from build123d import *

# Parameters (mm, degrees)
SKETCH1_W           = 15
SKETCH1_H           = 15
BOSS_EXTRUDE1_DEPTH = 10
BOSS_EXTRUDE2_DEPTH = 1.5


with BuildPart() as part:
    # Sketch1 → Boss-Extrude1 (new body)
    with BuildSketch(Plane.XY):
        with Locations((7.5, -7.5)):
            Rectangle(SKETCH1_W, SKETCH1_H)
    extrude(amount=BOSS_EXTRUDE1_DEPTH)

    # Sketch2 → Boss-Extrude2 (add, symmetric)
    with BuildSketch(Plane(origin=(7.5, 0, 0), x_dir=(0, 0, -1), z_dir=(1, 0, 0))):
        with BuildLine():
            ThreePointArc((3, -5), (0.5, -7.5), (3, -10))
            Line((3, -10), (3, -8.5))
            ThreePointArc((3, -8.5), (2, -7.5), (3, -6.5))
            Line((3, -6.5), (3, -5))
        make_face()
        with BuildLine():
            Line((3, -8.5), (3, -10))
            ThreePointArc((3, -10), (4.767766953, -9.267766953), (5.5, -7.5))
            ThreePointArc((5.5, -7.5), (4.767766953, -5.732233047), (3, -5))
            Line((3, -5), (3, -6.5))
            ThreePointArc((3, -6.5), (3.707106781, -6.792893219), (4, -7.5))
            ThreePointArc((4, -7.5), (3.707106781, -8.207106781), (3, -8.5))
        make_face()
        with BuildLine():
            Line((0, -10), (3, -10))
            ThreePointArc((3, -10), (0.5, -7.5), (3, -5))
            Line((3, -5), (0, -5))
            Line((0, -5), (0, -10))
        make_face()
    extrude(amount=BOSS_EXTRUDE2_DEPTH, both=True)


solid = part.part
Check sheet for the modelled part. Datum: model origin and axes. Units: mm. A direction names the side the tool comes from. Round coordinates to 2 decimals unless told otherwise and drop trailing zeros. Loops run counter-clockwise (first coordinate to the right, second up) from the corner with the lowest first, then second, coordinate; pieces in that order, holes last. Notation, with made-up numbers: (-9.75, 19.25) - (1.25, 19.25) arc R7 ccw to (1.25, 27.25) - close; hole circle Ø11 at (8.25, -9.5). An arc over 180 degrees is marked (long way). Answer as CSV lines item,"result". Start each with the question number.
Item 1: Section check B-B (z = -2.75). Record the boundary of the cut face in (x, y).
Item 2: Section check D-D (y = -14). Record the boundary of the cut face in (x, z).
Item 3: Section check A-A (x = 8.5). Record the boundary of the cut face in (y, z).
Item 4: Scan lines: line 1 (Z direction, x = 13.75, y = -4.75); line 2 (Y direction, x = 8, z = -2.5). Record each from-to range of solid material in increasing order. Write a range as [from, to].
Item 5: Section check C-C (y = -6.75). Record the boundary of the cut face in (x, z).
Item 6: Set-up check for faces 1 (the flat face through (9, -7, -1)), 2 (the flat face through (6, -7, -1)), 3 (the flat face through (8, -5, -2)), 4 (the flat face through (8, -10, -1)): record each of +Z, -Z, +X, -X, +Y, -Y from which the full face is reachable in a straight line by a thin tool's end or side.
Item 7: Depth check by flat-ended pin: P1, Ø1.5, axis at x = 7.5, z = -1, coming from the -Y side; P2, Ø6, axis at y = -6.5, z = -0.5, coming from the -X side; P3, Ø5.5, axis at y = -8, z = -4, coming from the -X side; P4, Ø2.5, axis at x = 7, z = -1.5, coming from the +Y side. Enter the tip coordinate at first touch or a pass-through.
Report:
1,outline,"(6, -10) - (9, -10) - (9, -8.47) - (6, -8.47) - close; (6, -6.53) - (9, -6.53) - (9, -5) - (6, -5) - close"
2,outline,"(0, 0) - (15, 0) - (15, 10) - (0, 10) - close"
3,outline,"(-15, 0) - (-10, 0) - (-10, -3) arc R2.5 ccw to (-5, -3) - (-5, 0) - (0, 0) - (0, 10) - (-15, 10) - close; hole circle Ø2 at (-7.5, -3)"
4,line 1,"z = [0, 10]"
4,line 2,"y = [-10, -8.37], [-6.63, -5]"
5,outline,"(0, 0) - (6, 0) - (6, -2.34) - (9, -2.34) - (9, 0) - (15, 0) - (15, 10) - (0, 10) - close; (6, -5.38) - (9, -5.38) - (9, -3.66) - (6, -3.66) - close"
6,face 1,"-Z, +X, +Y, -Y"
6,face 2,"-Z, -X, +Y, -Y"
6,face 3,"-Z, +X, -X, +Y"
6,face 4,"-Z, +X, -X, -Y"
7,P1,"stops at y = -10"
7,P2,"stops at x = 0"
7,P3,"stops at x = 6"
7,P4,"stops at y = -5"
